Check sheet for the drawn part. Datum: minimum x, y, z corner. Units: mm. Round coordinates to 2 decimals unless told otherwise and drop trailing zeros. Loops run counter-clockwise (first coordinate to the right, second up) from the corner with the lowest first, then second, coordinate; pieces in that order, holes last.
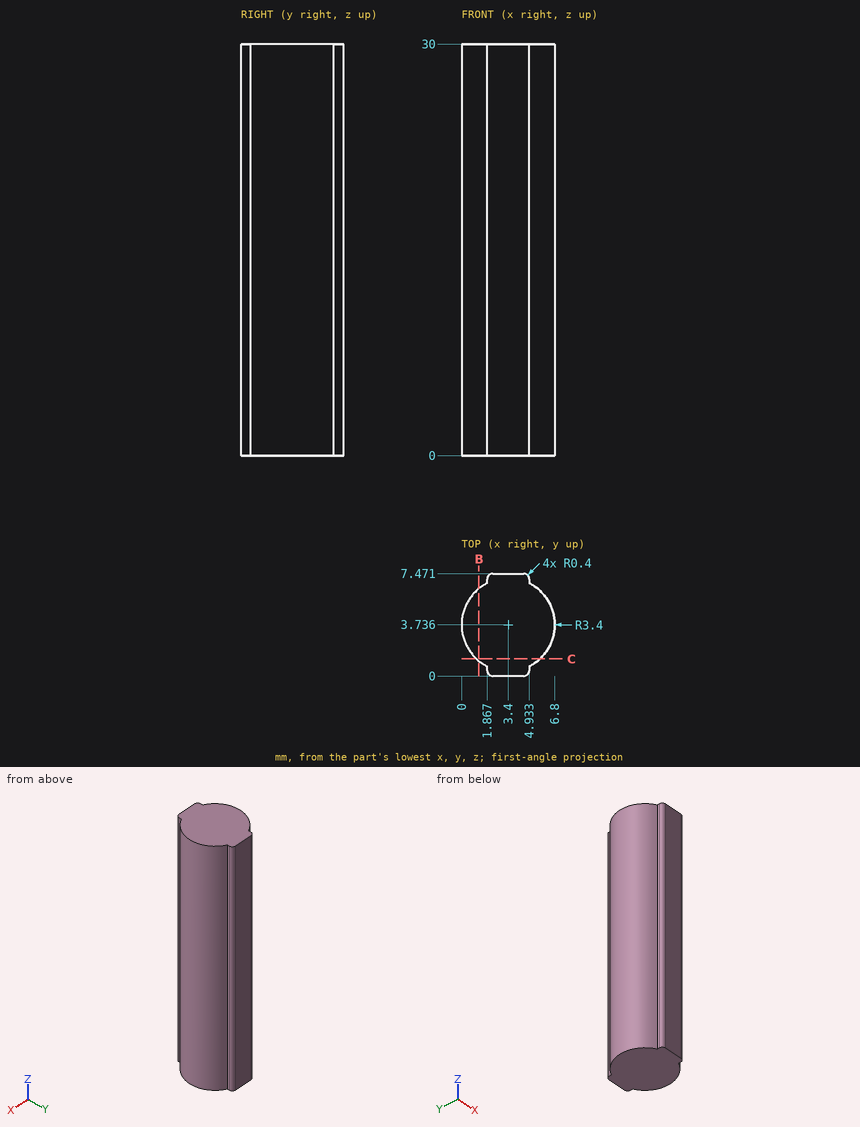
1. Section check B-B (x = 1.25). Enter the section's corners in (y, z).
2. Scan lines: L1, parallel to X at y = 7, z = 25; L2, parallel to X at y = 6, z = 12.5 (1 decimal); L3, parallel to Y at x = 1.5, z = 16.75 (1 decimal). Record each from-to range of solid material in increasing order.
3. Section check C-C (y = 1.25). Enter the section's corners in (x, z).
4. Gauge pin test, flat end, axial feed: P1, Ø2, axis at y = 6, z = 7.5, coming from the +X side. Record the tip position at first contact, or that the pin passes through.
Taken from the geometry:
1. outline: (1.1, 0) - (6.37, 0) - (6.37, 30) - (1.1, 30) - close
2. L1: x = 1.87 to 4.93
2. L2: x = 0.9 to 5.9
2. L3: y = 0.9 to 6.6
3. outline: (1.08, 0) - (5.72, 0) - (5.72, 30) - (1.08, 30) - close
4. P1: stops at x = 6.56
